from build123d import *

# Parameters (mm, degrees)
SKETCH3_R      = 0.25
EXTRUDE1_DEPTH = 8


with BuildPart() as part:
    # Sketch3 → Extrude1 (new body)
    with BuildSketch(Plane(origin=(0, 1, 0), x_dir=(1, 0, 0), z_dir=(0, 1, 0))):
        with Locations((-4.7, 0)):
            Circle(SKETCH3_R)
    extrude(amount=-EXTRUDE1_DEPTH)



with BuildPart() as body_2:
    # Sketch2 → Revolve-Thin1 (revolve)
    with BuildSketch(Plane(origin=(0, 0, 0), x_dir=(-1, 0, 0), z_dir=(0, 0, 1))):
        with BuildLine():
            Line((-3, 0), (-3, -0.75))
            ThreePointArc((-3, -0.75), (-2.926776695, -0.926776695), (-2.75, -1))
            Line((-2.75, -1), (0, -1))
            Line((0, -1), (0, -0.75))
            Line((0, -0.75), (-2.75, -0.75))
            Line((-2.75, -0.75), (-2.75, 0))
            Line((-2.75, 0), (-3, 0))
        make_face()
    revolve(axis=Axis((0, -0.05, 0), (0, 1, 0)))


with BuildPart() as part_1:
    add(part.part)

    add(body_2.part)  # Revolve-Thin2 merges body 2
    # Sketch1 → Revolve-Thin2 (revolve)
    with BuildSketch(Plane.XY):
        with BuildLine():
            Line((-4.5, 1), (-4.5, 0.25))
            ThreePointArc((-4.5, 0.25), (-4.426776695, 0.073223305), (-4.25, 0))
            Line((-4.25, 0), (-3.25, 0))
            ThreePointArc((-3.25, 0), (-3.073223305, 0.073223305), (-3, 0.25))
            Line((-3, 0.25), (-3, 1))
            Line((-3, 1), (-3.25, 1))
            Line((-3.25, 1), (-3.25, 0.25))
            Line((-3.25, 0.25), (-4.25, 0.25))
            Line((-4.25, 0.25), (-4.25, 1))
            Line((-4.25, 1), (-4.5, 1))
        make_face()
    revolve(axis=Axis((0, 1.05, 0), (0, -1, 0)))


solid = part_1.part
Check sheet for the modelled part. Datum: model origin and axes. Units: mm. A direction names the side the tool comes from. Give positions to 0.01 mm unless a question says otherwise; leave off trailing zeros. Loops run counter-clockwise (first coordinate to the right, second up) from the corner with the lowest first, then second, coordinate; pieces in that order, holes last. Notation, with made-up numbers: M 82,42.25 L 99,42.25 A21 ccw 99,69.25 Z; hole C 26.5,11 d11. An arc over 180 degrees is marked long. Answer as a JSON object with one key per item and string values. Group by question number.
Q1. Cross-section at C-C on x = -4.7. Record the cut outline in (y, z), then the cut area to 3 significant figures.
Q2. Access from +Z, -Z, +X, -X, +Y, -Y to the whole of each face (thin tool, end or side, straight path). Record for faces 3 (the cylindrical face through (2.579, 0.62, 1.978)), 4 (the cylindrical face through (-0.596, 0.37, 2.685)).
Q3. Material ranges on line 1 along X through (y, z) = (0.6, 0); line 2 along Z through (x, y) = (0, 0.6); line 3 along Y through (x, z) = (-1, 3.25), recorded low to high. Write a range as [from, to].
Q4. Cross-section at B-B on y = -2. Record the cut outline in (x, z), then the cut area to 3 significant figures.
Q5. Release check for a two-part mould opening along X. For faces 1 (the flat face through (0, 1, 0)), 2 (the cylindrical face through (-2.285, 0.63, -3.584)) record: released by +X, released by -X, zero draft, split by the parting line, or undercut.
Q6. Go/stop test with flat-tipped pins: P1, Ø1.6, axis at x = -1, z = 0.5, coming from the -Y side; P2, Ø2, axis at x = -1.5, y = 0, coming from the -Z side; P3, Ø2, axis at x = 2.5, y = -2, coming from the -Z side. Record where each tip stops, or that it passes through.
Evaluation:
{
 "1": {"outline": "M -7,-0.25 L 1,-0.25 L 1,0.25 L -7,0.25 Z", "area": "4.00 mm2"},
 "2": {"face 3": "+Y", "face 4": "-Y"},
 "3": {"line 1": "x = [-4.95, -4.25], [-3.25, -2.75], [2.75, 3.25], [4.25, 4.5]", "line 2": "z = [-4.5, -4.25], [-3.25, -2.75], [2.75, 3.25], [4.25, 4.5]", "line 3": "y = [0, 0.25]"},
 "4": {"outline": "C -4.7,0 d0.5", "area": "0.196 mm2"},
 "5": {"face 1": "zero draft", "face 2": "undercut"},
 "6": {"P1": "stops at y = 0.75", "P2": "stops at z = -4.47", "P3": "passes through"}
}
